from build123d import *

# Parameters (mm, degrees)
F1_DEPTH = 30
F2_DEPTH = 10


with BuildPart() as f1:
    # F0 (on Front) → F1 (new body)
    with BuildSketch(Plane.XZ):
        Polygon((-27.897622, 24.986569), (-33.67534, 21.23886), (-33.318587, 14.361355), (-27.184117, 11.23156), (-21.406399, 14.979269), (-21.763152, 21.856774), align=None)
        Polygon((-24.185025, 20.285829), (-23.977814, 16.2912), (-27.333658, 14.114435), (-30.896714, 15.9323), (-31.103926, 19.926929), (-27.748081, 22.103694), align=None, mode=Mode.SUBTRACT)
    extrude(amount=F1_DEPTH)

    # F0 (on Front) → F2 (join)
    with BuildSketch(Plane.XZ):
        Polygon((-27.333658, 14.114435), (-23.977814, 16.2912), (-24.185025, 20.285829), (-27.748081, 22.103694), (-31.103926, 19.926929), (-30.896714, 15.9323), align=None)
    extrude(amount=F2_DEPTH)


solid = f1.part
Geometry check sheet. Reference: the model listing, model coordinates, mm. A direction names the side the tool comes from. Give positions to 0.01 mm unless a question says otherwise; leave off trailing zeros. Loops run counter-clockwise (first coordinate to the right, second up) from the corner with the lowest first, then second, coordinate; pieces in that order, holes last. Notation, with made-up numbers: M 21,42.25 L 50,42.25 A23 cw 50,66.25 Z; hole C 46.5,5.5 d5. An arc over 180 degrees is marked long. Answer as a JSON object with one key per item and string values. Group by question number.
Item 1: Sectioned sample at A-A on y = -11. Record the boundary of the cut face in (x, z), plus the area to 3 significant figures.
Item 2: Material ranges on L1, parallel to Z at x = -25.5, y = -21.25; L2, parallel to Z at x = -30, y = -20.75; L3, parallel to Y at x = -28, z = 17.5, recorded low to high.
Item 3: Gauge pin test, flat ends, axial feed: pin 1 (2 mm diameter, centred on x = -28.5, z = 20, fed in from -Y); pin 2 (1 mm diameter, centred on x = -30, y = -20.5, fed in from -Z); pin 3 (3 mm diameter, centred on y = -20, z = 23, fed in from +X). Record the tip position at first contact, or that the pin passes through.
Item 4: Sectioned sample at C-C on y = -5. Record the boundary of the cut face in (x, z), plus the area to 3 significant figures.
Item 5: Sectioned sample at B-B on z = 20.75. Record the boundary of the cut face in (x, y), plus the area to 3 significant figures.
Item 6: Sectioned sample at D-D on x = -30.25. Record the boundary of the cut face in (y, z).
Item 7: Access from +Z, -Z, +X, -X, +Y, -Y to the whole of each face (thin tool, end or side, straight path). Record for faces 4 (the flat face through (-24.083, -19.86, 18.316)), 5 (the flat face through (-30.746, -14.79, 23.139)).
Item 8: Mould release check, pull along X, two halves, no side actions. Record for faces 1 (the flat face through (-25.63, -19.86, 15.22)), 2 (the flat face through (-25, -30, 15)), 3 (the flat face through (-21.582, -14.79, 18.37)): pulls with the +X half, pulls with the -X half, needs draft (parallel to the pull), parting line crosses it, or undercut.
Findings below:
{
 "1": {"outline": "M -33.68,21.24 L -33.32,14.36 L -27.18,11.23 L -21.41,14.98 L -21.76,21.86 L -27.9,24.99 Z; hole M -31.1,19.93 L -30.9,15.93 L -27.33,14.11 L -23.98,16.29 L -24.19,20.29 L -27.75,22.1 Z", "area": "81.7 mm2"},
 "2": {"L1": "12.32 to 15.3, 20.96 to 23.76", "L2": "12.67 to 15.47, 20.64 to 23.62", "L3": "-10 to 0"},
 "3": {"pin 1": "y = -10", "pin 2": "z = 12.41", "pin 3": "x = -21.74"},
 "4": {"outline": "M -33.68,21.24 L -33.32,14.36 L -27.18,11.23 L -21.41,14.98 L -21.76,21.86 L -27.9,24.99 Z", "area": "123 mm2"},
 "5": {"outline": "M -33.65,-30 L -29.84,-30 L -29.84,-10 L -25.09,-10 L -25.09,-30 L -21.71,-30 L -21.71,0 L -33.65,0 Z", "area": "264 mm2"},
 "6": {"outline": "M -30,12.8 L 0,12.8 L 0,23.46 L -30,23.46 L -30,20.48 L -10,20.48 L -10,15.6 L -30,15.6 Z"},
 "7": {"face 4": "-Y", "face 5": "+Z, -X, +Y, -Y"},
 "8": {"face 1": "undercut", "face 2": "needs draft", "face 3": "pulls with the +X half"}
}
